Verification items for the finished model (mm, model axes). A direction names the side the tool comes from. Give positions to 0.01 mm unless a question says otherwise; leave off trailing zeros. Loops run counter-clockwise (first coordinate to the right, second up) from the corner with the lowest first, then second, coordinate; pieces in that order, holes last. Notation, with made-up numbers: (84, 8.25) - (132, 8.25) arc R13 ccw to (132, 25.25) - close; hole circle Ø2 at (66, 58.25). An arc over 180 degrees is marked (long way). One line per item, written item: value. Start each with the question number.
1. Sectioned sample at D-D (x = 1). Record the cut outline in (y, z), plus the area to 3 significant figures.
2. Access from +Z, -Z, +X, -X, +Y, -Y to the whole of each face (thin tool, end or side, straight path). Record for faces 1 (the flat face through (0, 0, 0)), 2 (the cylindrical face through (3.9, 0.03, 0.75)), 3 (the flat face through (-7, -1.2, 2.2)).
3. Sectioned sample at A-A (z = 0). Record the cut outline in (x, y).
4. Gauge pin test, flat ends, axial feed: pin 1 (1 mm diameter, centred on x = -2.5, y = -2.5, fed in from +Z); pin 2 (0.8 mm diameter, centred on y = 0.5, z = 0, fed in from +X); pin 3 (6 mm diameter, centred on x = 1.5, z = 2.5, fed in from -Y). Record the tip position at first contact, or that the pin passes through.
5. Sectioned sample at C-C (x = 7). Record the cut outline in (y, z), plus the area to 3 significant figures.
6. Mould release check, pull along Z, two halves, no side actions. Record for faces 4 (the flat face through (7.5, 1, -1)), 5 (the cylindrical face through (-4, 0, -5)), 6 (the cylindrical face through (8.26, 1.917, -2.5)), 7 (the flat face through (9, 3, -2)): pulls with the +Z half, pulls with the -Z half, needs draft (parallel to the pull), parting line crosses it, or undercut.
7. Scan lines: L1, parallel to Y at x = -2.5, z = 0; L2, parallel to X at y = -0.5, z = -1; L3, parallel to Y at x = -4.25, z = 1. Record each from-to range of solid material in increasing order. Write a range as [from, to].
from build123d import *

# Parameters (mm, degrees)
SKIZZE2_R                       = 0.75
SCHNITT_LINEAR_AUSTRAGEN1_DEPTH = 17.132265805
AUFSATZ_LINEAR_START            = -0.2
SKIZZE3_R                       = 0.75
AUFSATZ_LINEAR_AUSTRAGEN1_DEPTH = 0.2


with BuildPart() as part:
    # Skizze1 → Rotation1 (revolve)
    with BuildSketch(Plane.XY, mode=Mode.PRIVATE) as rotation1_sk:
        Polygon((7.5, 0), (7.5, 3.15), (9, 3.15), (9, 4), (-1, 5), (-7, 5), (-7, 2.3), (0, 2.3), (0, 0), align=None)
    revolve(rotation1_sk.sketch.rotate(Axis((0, 0, 0), (1, 0, 0)), 90), axis=Axis((0, 0, 0), (1, 0, 0)))

    # Skizze2 → Schnitt-Linear austragen1 (cut, through all)
    with BuildSketch(Plane(origin=(7.5, 0, 0), x_dir=(0, 0, -1), z_dir=(1, 0, 0))):
        Circle(SKIZZE2_R)
    extrude(amount=-SCHNITT_LINEAR_AUSTRAGEN1_DEPTH, mode=Mode.SUBTRACT)

    # Skizze3 → Aufsatz-Linear austragen1 (add)
    with BuildSketch(Plane.ZY.offset(AUFSATZ_LINEAR_START)):
        with Locations(Location((0, 0, 0), (0, 0, 180))):
            Circle(SKIZZE3_R)
    extrude(amount=AUFSATZ_LINEAR_AUSTRAGEN1_DEPTH)


solid = part.part
Results are:
1. outline: circle Ø9.6 at (0, 0); hole circle Ø1.5 at (0, 0)
1. area: 70.6 mm^2
2. face 1: -X
2. face 2: +X
2. face 3: +Z, -Z, -X, +Y, -Y
3. outline: (-7, -5) - (-1, -5) - (9, -4) - (9, -3.15) - (7.5, -3.15) - (7.5, -0.75) - (0.2, -0.75) - (0.2, 0.75) - (7.5, 0.75) - (7.5, 3.15) - (9, 3.15) - (9, 4) - (-1, 5) - (-7, 5) - (-7, 2.3) - (0, 2.3) - (0, -2.3) - (-7, -2.3) - close
4. pin 1: stops at z = 4.58
4. pin 2: stops at x = 7.5
4. pin 3: stops at y = -4.95
5. outline: circle Ø8.4 at (0, 0); hole circle Ø1.5 at (0, 0)
5. area: 53.7 mm^2
6. face 4: undercut
6. face 5: parting line crosses it
6. face 6: undercut
6. face 7: needs draft
7. L1: y = [-5, -2.3], [2.3, 5]
7. L2: x = [0, 7.5]
7. L3: y = [-4.9, -2.07], [2.07, 4.9]
